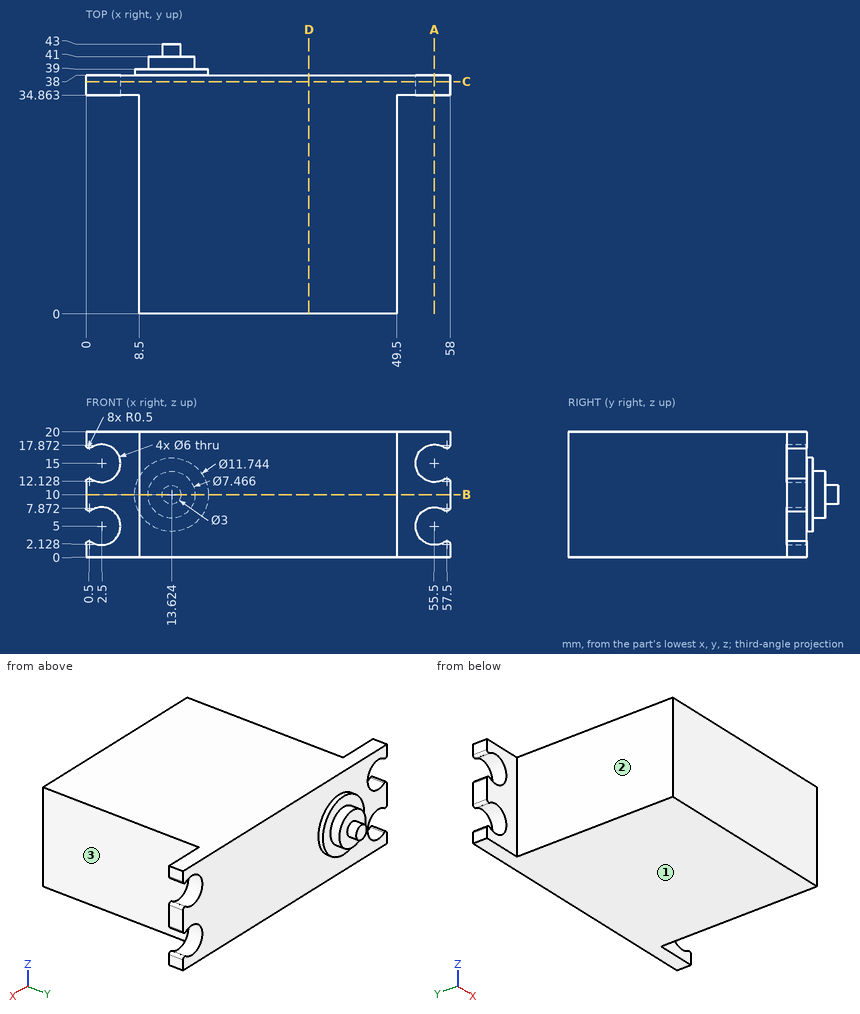
Input: dimensioned drawing with shaded views. Units: mm. Origin: part minimum x, y, z. A direction names the side the tool comes from. Give positions to 0.01 mm unless a question says otherwise; leave off trailing zeros. Order: outer loops, then holes, each group sorted by start corner. A loop starts at its lowest first (then second) coordinate and runs counter-clockwise, first axis right, second up.
(1) Section query B-B (z = 10). Return the cut outline in (x, y), plus the area to 3 significant figures.
(2) Material intervals for line 1 along Z through (x, y) = (55.5, 35.65); line 2 along X through (y, z) = (3, 2); line 3 along Y through (x, z) = (22.5, 18.25), sorted ascending.
(3) Contact query for flat-ended pins moving along their axis: P1, Ø1.5, axis at x = 52, z = 16.5, coming from the +Y side; P2, Ø7, axis at x = 54, z = 5, coming from the -Y side; P3, Ø4, axis at y = 17.5, z = 10.5, coming from the -X side. Output: stop coordinate, or through.
(4) Section query A-A (x = 55.5). Return the cut outline in (y, z).
(5) Access query for the marked faces 1, 2 and 3. Directions: +Z, -Z, +X, -X, +Y, -Y. A direction counts if a zero-diameter tool reaches every point of the face in a straight line with its end or side. Return the directions, or none.
(6) Section query C-C (y = 37). Return the cut outline in (x, z) (1 decimal), plus the area to 3 significant figures.
(7) Section query D-D (x = 35.5). Return the cut outline in (y, z).
Outcome:
1. outline: (0, 34.86) - (8.5, 34.86) - (8.5, 0) - (49.5, 0) - (49.5, 34.86) - (58, 34.86) - (58, 38) - (19.5, 38) - (19.5, 39) - (17.36, 39) - (17.36, 41) - (15.12, 41) - (15.12, 43) - (12.12, 43) - (12.12, 41) - (9.89, 41) - (9.89, 39) - (7.75, 39) - (7.75, 38) - (0, 38) - close
1. area: 1,640 mm2
2. line 1: z = 0 to 2, 8 to 12, 18 to 20
2. line 2: x = 8.5 to 49.5
2. line 3: y = 0 to 38
3. P1: stops at y = 38
3. P2: stops at y = 34.86
3. P3: stops at x = 8.5
4. outline: (34.86, 0) - (38, 0) - (38, 2) - (34.86, 2) - close; (34.86, 8) - (38, 8) - (38, 12) - (34.86, 12) - close; (34.86, 18) - (38, 18) - (38, 20) - (34.86, 20) - close
5. face 1: -Z, +X, -X, +Y, -Y
5. face 2: +Z, -Z, -X, -Y
5. face 3: +Z, -Z, +X, -Y
6. outline: (0, 0) - (58, 0) - (58, 2.1) arc R0.5 ccw to (57.2, 2.5) arc R3 cw (long way) to (57.2, 7.5) arc R0.5 ccw to (58, 7.9) - (58, 12.1) arc R0.5 ccw to (57.2, 12.5) arc R3 cw (long way) to (57.2, 17.5) arc R0.5 ccw to (58, 17.9) - (58, 20) - (0, 20) - (0, 17.9) arc R0.5 ccw to (0.8, 17.5) arc R3 cw (long way) to (0.8, 12.5) arc R0.5 ccw to (0, 12.1) - (0, 7.9) arc R0.5 ccw to (0.8, 7.5) arc R3 cw (long way) to (0.8, 2.5) arc R0.5 ccw to (0, 2.1) - close
6. area: 1,050 mm2
7. outline: (0, 0) - (38, 0) - (38, 20) - (0, 20) - close
